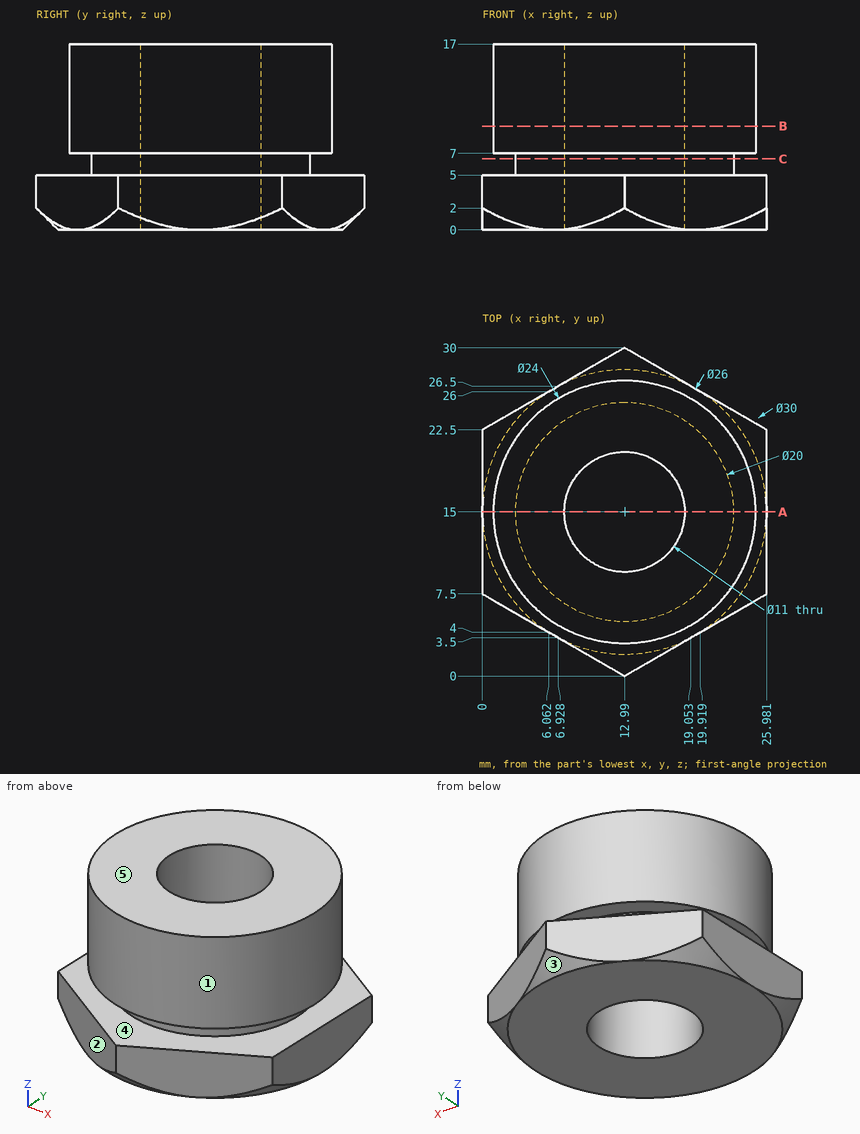
Here's the drawing with two shaded views (mm, measured from the low corner). I have some questions. A direction names the side the tool comes from. Coordinates: 2 decimals unless noted, no trailing zeros. Write each loop counter-clockwise with the first axis right and the second up, starting at its lowest first coordinate (ties: lowest second). Pieces come first, ordered by that corner, then holes. Notation, with made-up numbers: (75.25, 87.25) -> (88.25, 87.25) arc R9 ccw to (88.25, 102.25) -> close; hole circle Ø10 at (-22.75, -39.75). An arc over 180 degrees is marked (long way). Write item = value, one per line. Start each with the question number.
(1) Which directions (+Z, -Z, +X, -X, +Y, -Y) give clear straight access to the entire face, cutting with the end or side of a thin tool? Please do the marked faces 1 and 2.
(2) We'd pull the mould along Z, two halves only. Please class the marked faces 3, 4 and 5: released by +Z, released by -Z, zero draft, split by the parting line, or undercut.
(3) I want a section at A-A (y = 15). Please give me the cut outline in (x, z).
(4) I need wall thicknesses on line 1 (Z direction, x = 12, y = 3.5); line 2 (X direction, y = 13, z = 14.5) (1 decimal); line 3 (Y direction, x = 9.5, z = 10.25). Which ranges of each line are inside material? Lowest first, please. Write a range as [from, to].
(5) Will these pins go through, and if not, where does the flat tip stop? pin 1 (1.5 mm diameter, centred on x = 4, z = 8, fed in from +Y) (1 decimal); pin 2 (10 mm diameter, centred on x = 14, z = 14.5, fed in from -Y); pin 3 (10 mm diameter, centred on x = 19.5, z = 6.5, fed in from +Y) (1 decimal).
(6) I want a section at C-C (z = 6.5). Please give me the cut outline in (x, y).
(7) I want a section at B-B (z = 9.5). Please give me the cut outline in (x, y).
Result set:
q1.face_1 = +Z
q1.face_2 = +Z, -Z, -X, -Y
q2.face_3 = released by -Z
q2.face_4 = undercut
q2.face_5 = released by +Z
q3.outline = (0, 0) -> (7.49, 0) -> (7.49, 17) -> (0.99, 17) -> (0.99, 7) -> (2.99, 7) -> (2.99, 5) -> (0, 5) -> close; (18.49, 0) -> (25.98, 0) -> (25.98, 5) -> (22.99, 5) -> (22.99, 7) -> (24.99, 7) -> (24.99, 17) -> (18.49, 17) -> close
q4.line_1 = [0, 5], [7, 17]
q4.line_2 = [1.2, 7.9], [18.1, 24.8]
q4.line_3 = [3.52, 10.75], [19.25, 26.48]
q5.pin_1 = 23.7
q5.pin_2 = 3
q5.pin_3 = 29
q6.outline = circle Ø20 at (12.99, 15); hole circle Ø11 at (12.99, 15)
q7.outline = circle Ø24 at (12.99, 15); hole circle Ø11 at (12.99, 15)
